Can you work these out from the model? Positions are in its coordinate system, mm. A direction names the side the tool comes from. Round coordinates to 2 decimals unless told otherwise and drop trailing zeros. Loops run counter-clockwise (first coordinate to the right, second up) from the corner with the lowest first, then second, coordinate; pieces in that order, holes last. Notation, with made-up numbers: (-16, -16) -> (-5, -16) arc R18 ccw to (-5, -8) -> close; hole circle Ø10 at (43, 12.5). An arc over 180 degrees is marked (long way). Answer as a JSON object with one key per item and string values.
Autodesk Inventor part; units mm, degrees
ref_plane "YZ Plane" through (0, 0, 0) normal (1, 0, 0) x (0, 1, 0)
ref_plane "XZ Plane" through (0, 0, 0) normal (0, 1, 0) x (-1, 0, 0)
ref_plane "XY Plane" through (0, 0, 0) normal (0, 0, 1) x (1, 0, 0)
sketch "Skizze2" plane through (0, 0, 0) normal (0, 0, 1) x (1, 0, 0)
  line L0 (0, 0) -> (23, 0)
  line L1 (23, 0) -> (23, 18)
  line L2 (23, 18) -> (3, 18)
  line L3 (0, 6) -> (0, 0)
  line L4 (0, 0) -> (0, 6)
  line L5 (0, 6) -> (3, 6)
  line L6 (3, 6) -> (3, 18)
  line L7 (0, 6) -> (3, 9)
  line L8 (0, 0) -> (19.6, 0)
  line L9 (19.6, 0) -> (19.6, 6.8)
  line L10 (23, 0) -> (23, 12)
  line L11 (9.5, 0) -> (9.5, 11.8)
  line L12 (14, 14) -> (23, 14)
  line L13 (14, 14) -> (14, 18)
  dimension "d21" = 18
  dimension "d22" = 6
  dimension "d23" = 3
  dimension "d24" = 23
  dimension "d25" = 45
  dimension "d26" = 19.6
  dimension "d27" = 6.8
  dimension "d28" = 12
  dimension "d30" = 11.8
  dimension "d31" = 9.5
  dimension "d36" = 14
  dimension "d37" = 9
extrude "Extrusion1" add sketch "Skizze2" along normal mid plane 6 contours L3 L5 L6 L2 L13 L12 L1 L0 | L7 L6 L5
hole "Bohrung1" at (19.6, 6.8, 0) at (9.5, 11.8, 0) direction (0, 0, -1) diameter 4 end through all both
fillet "Rundung1" radius 3 4 edges at (0, 6, 0) (3, 9, 0) (23, 14, 0) (14, 14, 0)
fillet "Rundung2" radius 4 1 edges at (3, 18, 0)
fillet "Rundung3" radius 3 1 edges at (14, 18, 0)
sketch "Skizze3" plane through (0, 0, 3) normal (0, -1, 0) x (1, 0, 0)
  line L0 (0, -3) -> (3.5, -3) construction
  line L1 (3.5, -3) -> (10.5, -3) construction
  line L2 (10.5, -3) -> (17.5, -3) construction
  dimension "d50" = 3.5
  dimension "d51" = 7
  dimension "d52" = 7
hole "Bohrung2" at (3.5, 0, 0) at (10.5, 0, 0) direction (0, 1, 0) diameter 2.459 depth 7 tip angle 118
hole "Bohrung3" at (17.5, 0, 0) direction (0, 1, 0) diameter 2.459 depth 4 tip angle 118
sketch "Skizze4" plane through (0, 0, 3) normal (0, 0, 1) x (1, 0, 0)
  line L0 (14, 0) -> (14, 2.5)
  line L1 (20.75, 0) -> (20.75, 2.5)
  line L2 (0, 4.7574) -> (0, 0)
  line L3 (0, 0) -> (0, 4.7574)
  point P0 (23, 0)
  dimension "d71" = 2.5
  dimension "d72" = 2.5
  dimension "d89" = 14
  dimension "d90" = 6.75
hole "Bohrung4" at (14, 2.5, 3) at (20.75, 2.5, 3) direction (0, 0, -1) diameter 2 end through all
sketch "Skizze5" plane through (0, 0, 3) normal (0, 0, 1) x (1, 0, 0)
  line L0 (20, 0) -> (20, 12)
  line L1 (0, 4.7574) -> (0, 0)
  line L2 (0, 0) -> (0, 4.7574)
  dimension "d81" = 12
  dimension "d91" = 20
hole "Bohrung5" at (20, 12, 3) direction (0, 0, -1) diameter 1.567 depth 6
properties part number "Lagerblock Dribbler"
Q1. I want a section at B-B, the plane z = 1.75. Give the number of separate pieces and of enclosed holes in the cut face, then the cut area to 3 significant figures.
Determined:
{"separate pieces": "1", "enclosed holes": "5", "area": "308 mm²"}
Q2. I want a section at A-A, the plane y = 5.25. Write out the boundary of the cut face in (x, z).
Determined:
{"outline": "(0.04, -3) -> (18.34, -3) -> (18.34, 3) -> (0.04, 3) -> close; (20.86, -3) -> (23, -3) -> (23, 3) -> (20.86, 3) -> close; hole circle Ø2.46 at (3.5, 0); hole circle Ø2.46 at (10.5, 0)"}
Q3. I want a section at D-D, the plane x = 1.5. Write out the boundary of the cut face in (y, z).
Determined:
{"outline": "(0, -3) -> (7.5, -3) -> (7.5, 3) -> (0, 3) -> close"}
Q4. I want a section at C-C, the plane y = 13.5. Write out the boundary of the cut face in (x, z).
Determined:
{"outline": "(3, -3) -> (8.45, -3) -> (8.45, 3) -> (3, 3) -> close; (10.55, -3) -> (21.66, -3) -> (21.66, 3) -> (10.55, 3) -> close"}
Q5. On a 3-axis mill with a long thin cutter (end or side, diameter ignored), from which of +Z, -Z, +X, -X, +Y, -Y can I reach the whole of each face in a straight line? I mean faces 1 (the flat face through (9, 18, 0)), 2 (the flat face through (3, 12, 0)), 3 (the cylindrical face through (16.28, 2.03, 0.16)). Say none if no direction works.
Determined:
{"face 1": "+Z, -Z, +X, -X, +Y", "face 2": "+Z, -Z, -X, +Y", "face 3": "-Y"}
Q6. If I drill on L1, parallel to X at y = 5.5, z = 0; L2, parallel to Z at x = 3.5, y = 3; L3, parallel to X at y = 6.8, z = -0.5, over which ranges is the centre line in solid material (lowest first)? Write a range as [from, to].
Determined:
{"L1": "[0.09, 2.27], [4.73, 9.27], [11.73, 18.08], [21.12, 23]", "L2": "[-3, -1.23], [1.23, 3]", "L3": "[0.8, 2.38], [4.62, 9.38], [11.62, 17.6], [21.6, 23]"}
Q7. We'd pull the mould along Y, two halves only. Please class faces 4 (the cylindrical face through (19.34, 11.58, -0.04)), 5 (the cylindrical face through (4.7, 3.55, 0.27)), 6 (the cylindrical face through (22.14, 13.1, 0.04)): pulls with the +Y half, pulls with the -Y half, needs draft (parallel to the pull), parting line crosses it, or undercut.
Determined:
{"face 4": "undercut", "face 5": "needs draft", "face 6": "pulls with the +Y half"}
Q8. I'm going to push flat-ended pins straight in: pin 1 (1.5 mm diameter, centred on x = 18, z = 0, fed in from +Y); pin 2 (3 mm diameter, centred on y = 13, z = -0.5, fed in from -X). Where does each tip first touch, or does it pass through?
Determined:
{"pin 1": "y = 14", "pin 2": "x = 3"}
